```python
from build123d import *

# Parameters (mm, degrees)
F1_DEPTH = 12.7


with BuildPart() as f1:
    # F0 (on Top) → F1 (new body, symmetric)
    with BuildSketch(Plane.XY):
        with BuildLine():
            Line((12.7, 0), (76.2, 0))
            ThreePointArc((76.2, 0), (75.933086, 6.372321), (75.134213, 12.7))
            ThreePointArc((75.134213, 12.7), (53.881537, 53.881537), (12.7, 75.134213))
            ThreePointArc((12.7, 75.134213), (6.372321, 75.933086), (0, 76.2))
            Line((0, 76.2), (0, 12.7))
            ThreePointArc((0, 12.7), (4.86008, 11.73327), (8.980256, 8.980256))
            ThreePointArc((8.980256, 8.980256), (11.73327, 4.86008), (12.7, 0))
        make_face()
        with BuildLine():
            ThreePointArc((19.05, 12.7), (14.559872, 14.559872), (12.7, 19.05))
            Line((12.7, 19.05), (12.7, 53.881537))
            ThreePointArc((12.7, 53.881537), (15.383826, 59.06629), (21.166667, 59.868374))
            ThreePointArc((21.166667, 59.868374), (44.901281, 44.901281), (59.868374, 21.166667))
            ThreePointArc((59.868374, 21.166667), (59.06629, 15.383826), (53.881537, 12.7))
            Line((53.881537, 12.7), (19.05, 12.7))
        make_face(mode=Mode.SUBTRACT)
        with BuildLine():
            ThreePointArc((75.134213, -12.7), (75.933086, -6.372321), (76.2, 0))
            Line((76.2, 0), (12.7, 0))
            ThreePointArc((12.7, 0), (11.73327, -4.86008), (8.980256, -8.980256))
            ThreePointArc((8.980256, -8.980256), (4.86008, -11.73327), (0, -12.7))
            Line((0, -12.7), (0, -76.2))
            ThreePointArc((0, -76.2), (6.372321, -75.933086), (12.7, -75.134213))
            ThreePointArc((12.7, -75.134213), (53.881537, -53.881537), (75.134213, -12.7))
        make_face()
        with BuildLine():
            ThreePointArc((12.7, -19.05), (14.559872, -14.559872), (19.05, -12.7))
            Line((19.05, -12.7), (53.881537, -12.7))
            ThreePointArc((53.881537, -12.7), (59.06629, -15.383826), (59.868374, -21.166667))
            ThreePointArc((59.868374, -21.166667), (44.901281, -44.901281), (21.166667, -59.868374))
            ThreePointArc((21.166667, -59.868374), (15.383826, -59.06629), (12.7, -53.881537))
            Line((12.7, -53.881537), (12.7, -19.05))
        make_face(mode=Mode.SUBTRACT)
        with BuildLine():
            Line((0, 12.7), (0, 76.2))
            ThreePointArc((0, 76.2), (-6.372321, 75.933086), (-12.7, 75.134213))
            ThreePointArc((-12.7, 75.134213), (-53.881537, 53.881537), (-75.134213, 12.7))
            ThreePointArc((-75.134213, 12.7), (-75.933086, 6.372321), (-76.2, 0))
            Line((-76.2, 0), (-12.7, 0))
            ThreePointArc((-12.7, 0), (-11.73327, 4.86008), (-8.980256, 8.980256))
            ThreePointArc((-8.980256, 8.980256), (-4.86008, 11.73327), (0, 12.7))
        make_face()
        with BuildLine():
            Line((-12.7, 53.881537), (-12.7, 19.05))
            ThreePointArc((-12.7, 19.05), (-14.559872, 14.559872), (-19.05, 12.7))
            Line((-19.05, 12.7), (-53.881537, 12.7))
            ThreePointArc((-53.881537, 12.7), (-59.06629, 15.383826), (-59.868374, 21.166667))
            ThreePointArc((-59.868374, 21.166667), (-44.901281, 44.901281), (-21.166667, 59.868374))
            ThreePointArc((-21.166667, 59.868374), (-15.383826, 59.06629), (-12.7, 53.881537))
        make_face(mode=Mode.SUBTRACT)
        with BuildLine():
            ThreePointArc((-12.7, -75.134213), (-6.372321, -75.933086), (0, -76.2))
            Line((0, -76.2), (0, -12.7))
            ThreePointArc((0, -12.7), (-4.86008, -11.73327), (-8.980256, -8.980256))
            ThreePointArc((-8.980256, -8.980256), (-11.73327, -4.86008), (-12.7, 0))
            Line((-12.7, 0), (-76.2, 0))
            ThreePointArc((-76.2, 0), (-75.933086, -6.372321), (-75.134213, -12.7))
            ThreePointArc((-75.134213, -12.7), (-53.881537, -53.881537), (-12.7, -75.134213))
        make_face()
        with BuildLine():
            ThreePointArc((-21.166667, -59.868374), (-44.901281, -44.901281), (-59.868374, -21.166667))
            ThreePointArc((-59.868374, -21.166667), (-59.06629, -15.383826), (-53.881537, -12.7))
            Line((-53.881537, -12.7), (-19.05, -12.7))
            ThreePointArc((-19.05, -12.7), (-14.559872, -14.559872), (-12.7, -19.05))
            Line((-12.7, -19.05), (-12.7, -53.881537))
            ThreePointArc((-12.7, -53.881537), (-15.383826, -59.06629), (-21.166667, -59.868374))
        make_face(mode=Mode.SUBTRACT)
    extrude(amount=F1_DEPTH, both=True)


solid = f1.part
```
Verification items for the finished model (mm, model axes). Give positions to 0.01 mm unless a question says otherwise; leave off trailing zeros. Loops run counter-clockwise (first coordinate to the right, second up) from the corner with the lowest first, then second, coordinate; pieces in that order, holes last.
1. Go/stop test with flat-tipped pins: pin 1 Ø12 at (y, z) = (-11.5, -7.5) entering from -X; pin 2 Ø10 at (y, z) = (40.5, 8) entering from -X; pin 3 Ø12.5 at (x, z) = (-36, -5) entering from +Y; pin 4 Ø10 at (y, z) = (-2, 0.5) entering from +X. Record where each tip stops, or that it passes through.
2. Section check C-C, the plane z = 8.25. Count the separate pieces of the cut face and the enclosed holes in it, then the cut area to 3 significant figures.
3. Section check A-A, the plane x = 32. Enter the section's corners in (y, z).
4. Section check B-B, the plane y = 56. Enter the section's corners in (x, z).
5. Section check D-D, the plane x = -62. Enter the section's corners in (y, z), then the cut area to 3 significant figures.
6. Thickness scan on line 1 (X direction, y = -37.5, z = 3.75); line 2 (X direction, y = -40.5, z = -8.75); line 3 (Y direction, x = 38, z = -5.75). Record the ranges inside material, lowest first.
7. Mould release check, pull along X, two halves, no side actions. Record for faces 1 (the cylindrical face through (53.41, -54.35, 0.18)), 2 (the flat face through (-1, -16, -12.7)), 3 (the cylindrical face through (59.017, -15.315, 0.178)): released by +X, released by -X, zero draft, split by the parting line, or undercut.
Geometry says:
1. pin 1: stops at x = -76
1. pin 2: stops at x = -67.43
1. pin 3: stops at y = 70.15
1. pin 4: stops at x = 76.2
2. separate pieces: 1
2. enclosed holes: 5
2. area: 11,000 mm2
3. outline: (-69.16, -12.7) - (-54.85, -12.7) - (-54.85, 12.7) - (-69.16, 12.7) - close; (-12.7, -12.7) - (12.7, -12.7) - (12.7, 12.7) - (-12.7, 12.7) - close; (54.85, -12.7) - (69.16, -12.7) - (69.16, 12.7) - (54.85, 12.7) - close
4. outline: (-51.68, -12.7) - (-29.94, -12.7) - (-29.94, 12.7) - (-51.68, 12.7) - close; (-13.06, -12.7) - (13.06, -12.7) - (13.06, 12.7) - (-13.06, 12.7) - close; (29.94, -12.7) - (51.68, -12.7) - (51.68, 12.7) - (29.94, 12.7) - close
5. outline: (-44.3, -12.7) - (44.3, -12.7) - (44.3, 12.7) - (-44.3, 12.7) - close
5. area: 2,250 mm2
6. line 1: x = -66.33 to -51.24, -12.7 to 12.7, 51.24 to 66.33
6. line 2: x = -64.55 to -48.91, -12.7 to 12.7, 48.91 to 64.55
6. line 3: y = -66.05 to -50.87, -12.7 to 12.7, 50.87 to 66.05
7. face 1: released by +X
7. face 2: zero draft
7. face 3: undercut
